Source: CAD feature listing. Evaluate the final solid. Frame: model axes, mm. Face numbers are marked on the shaded views. A direction names the side the tool comes from. Round coordinates to 2 decimals unless told otherwise and drop trailing zeros. Loops run counter-clockwise (first coordinate to the right, second up) from the corner with the lowest first, then second, coordinate; pieces in that order, holes last. Notation, with made-up numbers: (46.25, -20) - (64.25, -20) arc R17 ccw to (64.25, 1) - close; hole circle Ø1 at (-34, 28). An arc over 180 degrees is marked (long way). One line per question, with ' | ' between items. Start each with the question number.
1. Cut plane D-D (x = 0). State how many separate pieces and enclosed holes the cut face has, then the cut area to 3 significant figures.
2. Cut plane C-C (x = 4.5). Return loops of the section in (y, z) (3 decimals).
3. Ray query, line 1 (Y direction, x = 0, z = 0.2) (3 decimals); line 2 (Z direction, x = -8.5, y = -5.5); line 3 (X direction, y = -5, z = -5.25). Return the intervals inside material, ascending.
4. Cut plane B-B (z = -8.5). Return loops of the section in (x, y) (3 decimals).
5. Access query for the marked faces 5, 6 and 7. Directions: +Z, -Z, +X, -X, +Y, -Y. A direction counts if a zero-diameter tool reaches every point of the face in a straight line with its end or side. Return the directions, or none.
6. Pin query (flat end, axial travel): pin 1 (2 mm diameter, centred on y = 3, z = -6.5, fed in from -X); pin 2 (4 mm diameter, centred on x = -6, z = -10.5, fed in from -Y) (3 decimals); pin 3 (0.9 mm diameter, centred on x = -6.5, z = 0.5, fed in from +Y) (3 decimals). Return the tip coordinate at first contact, or that it passes through.
7. Mould query, pull axis Z, two halves, no side actions, for the marked faces 1, 2, 3 and 4. Classes: pulls with the +Z half, pulls with the -Z half, needs draft (parallel to the pull), parting line crosses it, or undercut.
8. Cut plane A-A (y = -2). Return loops of the section in (x, z), then the cut area to 3 significant figures.
Autodesk Inventor part; units mm, degrees
ref_plane "YZ Plane" through (0, 0, 0) normal (1, 0, 0) x (0, 1, 0)
ref_plane "XZ Plane" through (0, 0, 0) normal (0, 1, 0) x (-1, 0, 0)
ref_plane "XY Plane" through (0, 0, 0) normal (0, 0, 1) x (1, 0, 0)
sketch "Sketch1" plane through (0, 0, 0) normal (0, 0, 1) x (1, 0, 0)
  line L0 (-6.2, 6.875) -> (6.2, 6.875)
  line L1 (6.2, 6.875) -> (6.2, -6.875)
  line L2 (6.2, -6.875) -> (-6.2, -6.875)
  line L3 (-6.2, -6.875) -> (-6.2, 6.875)
  line L4 (8.8, 12.475) -> (-8.8, 12.475)
  line L5 (-11.8, 9.475) -> (-11.8, -9.475)
  line L6 (-8.8, -12.475) -> (8.8, -12.475)
  line L7 (11.8, -9.475) -> (11.8, 9.475)
  arc A0 (-8.8, 12.475) -> (-11.8, 9.475) centre (-8.8, 9.475) ccw
  arc A1 (11.8, 9.475) -> (8.8, 12.475) centre (8.8, 9.475) ccw
  arc A2 (8.8, -12.475) -> (11.8, -9.475) centre (8.8, -9.475) ccw
  arc A3 (-11.8, -9.475) -> (-8.8, -12.475) centre (-8.8, -9.475) ccw
  point P0 (0, 0)
  dimension "d0" = 12.4
  dimension "d1" = 13.75
  dimension "d2" = 5.6
  dimension "d3" = 3
  dimension "d4" = 6.875
  dimension "d5" = 6.2
  dimension "d16" = 23.6
  dimension "d17" = 24.95
extrude "Extrusion1" add sketch "Sketch1" along normal blind 0.8
sketch "Sketch3" plane through (0, 0, 0) normal (0, 0, -1) x (-1, 0, 0)
  line L0 (-6.2, -6.875) -> (-6.2, 6.875)
  line L1 (-6.2, 6.875) -> (6.2, 6.875)
  line L2 (6.2, 6.875) -> (6.2, -6.875)
  line L3 (6.2, -6.875) -> (-6.2, -6.875)
  line L4 (8.8, 12.475) -> (-8.8, 12.475)
  arc A0 (-8.8, 12.475) -> (-11.8, 9.475) centre (-8.8, 9.475) ccw
  line L5 (-11.8, 9.475) -> (-11.8, -9.475)
  arc A1 (-11.8, -9.475) -> (-8.8, -12.475) centre (-8.8, -9.475) ccw
  line L6 (-8.8, -12.475) -> (8.8, -12.475)
  arc A2 (8.8, -12.475) -> (11.8, -9.475) centre (8.8, -9.475) ccw
  line L7 (11.8, -9.475) -> (11.8, 9.475)
  arc A3 (11.8, 9.475) -> (8.8, 12.475) centre (8.8, 9.475) ccw
  line L8 (7, -7.675) -> (7, 7.675)
  line L9 (7, 7.675) -> (-7, 7.675)
  line L10 (-7, 7.675) -> (-7, -7.675)
  line L11 (-7, -7.675) -> (7, -7.675)
  point P0 (0, 0)
  dimension "d11" = 0.8
extrude "Extrusion2" add sketch "Sketch3" along normal blind 15 contours L11 L10 L9 L8
sketch "Sketch4" plane through (0, 0, -15) normal (0, 0, -1) x (-1, 0, 0)
  line L0 (7, -7.675) -> (-7, -7.675)
  line L1 (-7, -7.675) -> (-7, 7.675)
  line L2 (-7, 7.675) -> (7, 7.675)
  line L3 (7, 7.675) -> (7, -7.675)
  line L4 (8.8, 12.475) -> (-8.8, 12.475)
  arc A0 (-8.8, 12.475) -> (-11.8, 9.475) centre (-8.8, 9.475) ccw
  line L5 (-11.8, 9.475) -> (-11.8, -9.475)
  arc A1 (-11.8, -9.475) -> (-8.8, -12.475) centre (-8.8, -9.475) ccw
  line L6 (-8.8, -12.475) -> (8.8, -12.475)
  arc A2 (8.8, -12.475) -> (11.8, -9.475) centre (8.8, -9.475) ccw
  line L7 (11.8, -9.475) -> (11.8, 9.475)
  arc A3 (11.8, 9.475) -> (8.8, 12.475) centre (8.8, 9.475) ccw
  line L8 (-6.2, 6.875) -> (6.2, 6.875)
  line L9 (6.2, 6.875) -> (6.2, -6.875)
  line L10 (6.2, -6.875) -> (-6.2, -6.875)
  line L11 (-6.2, -6.875) -> (-6.2, 6.875)
  line L12 (7, -7.675) -> (7, 7.675)
  line L13 (7, 7.675) -> (-7, 7.675)
  line L14 (-7, 7.675) -> (-7, -7.675)
  line L15 (-7, -7.675) -> (7, -7.675)
  point P0 (0, 0)
extrude "Extrusion3" add sketch "Sketch4" along normal blind 0.8 contours L0 L1 L2 L3 | A3 L7 A2 L6 A1 L5 A0 L4
chamfer "Chamfer1" distance 1.1 angle 45 8 edges at (7, 0, 0) (0, -7.675, 0) (0, 7.675, 0) (-7, 0, 0) (-7, 0, -15) (0, 7.675, -15) (0, -7.675, -15) (7, 0, -15)
sketch "Sketch5" plane through (0, 0, 0.8) normal (0, 0, 1) x (1, 0, 0)
  circle A0 centre (0, 8.375) radius 0.6
  line L0 (-6.2, 6.875) -> (6.2, 6.875)
  line L1 (11.8, -9.475) -> (11.8, 9.475)
  line L2 (-11.8, 9.475) -> (-11.8, -9.475)
  line L3 (6.2, 6.875) -> (6.2, -6.875)
  line L4 (6.2, -6.875) -> (-6.2, -6.875)
  line L5 (-6.2, -6.875) -> (-6.2, 6.875)
  line L6 (-6.2, 6.875) -> (6.2, 6.875)
  line L7 (8.8, 12.475) -> (-8.8, 12.475)
  arc A1 (-8.8, 12.475) -> (-11.8, 9.475) centre (-8.8, 9.475) ccw
  line L8 (-11.8, 9.475) -> (-11.8, -9.475)
  arc A2 (-11.8, -9.475) -> (-8.8, -12.475) centre (-8.8, -9.475) ccw
  line L9 (-8.8, -12.475) -> (8.8, -12.475)
  arc A3 (8.8, -12.475) -> (11.8, -9.475) centre (8.8, -9.475) ccw
  line L10 (11.8, -9.475) -> (11.8, 9.475)
  arc A4 (11.8, 9.475) -> (8.8, 12.475) centre (8.8, 9.475) ccw
  line L11 (-8.8, 12.475) -> (8.8, 12.475)
  line L12 (3, 12.475) -> (-3, 12.475)
  line L13 (-3, 12.475) -> (-3, 19.475)
  line L14 (-3, 19.475) -> (3, 19.475)
  line L15 (3, 19.475) -> (3, 12.475)
  circle A5 centre (0, 11.375) radius 0.6
  circle A6 centre (0, 14.375) radius 0.6
  circle A7 centre (0, 17.375) radius 0.6
  point P0 (0, 0)
  dimension "d21" = 1.2
  dimension "d22" = 1.5
  dimension "d23" = 11.8
  dimension "d24" = 23.6
  dimension "d27" = 6
  dimension "d28" = 7
  dimension "d29" = 8.8
  dimension "d32" = 3
extrude "Extrusion4" add sketch "Sketch5" against normal up to surface (0.8 mm away) contours L7 L13 L14 L15
chamfer "Chamfer2" distance 2 angle 45 2 edges at (-3, 12.475, 0.4) (3, 12.475, 0.4)
extrude "Extrusion5" cut sketch "Sketch5" against normal blind 10 contours A0 | A5
fillet "Fillet1" radius 1 2 edges at (-3, 19.475, 0.4) (3, 19.475, 0.4)
equation "\"d23\" = 0.5 * d24"
equation "\"d29\" = -0.5 * d27 + 0.5 * d24"
properties part number "3DP_ABS_Electromagnet_Coil_Holder" material "ABS Plastic"
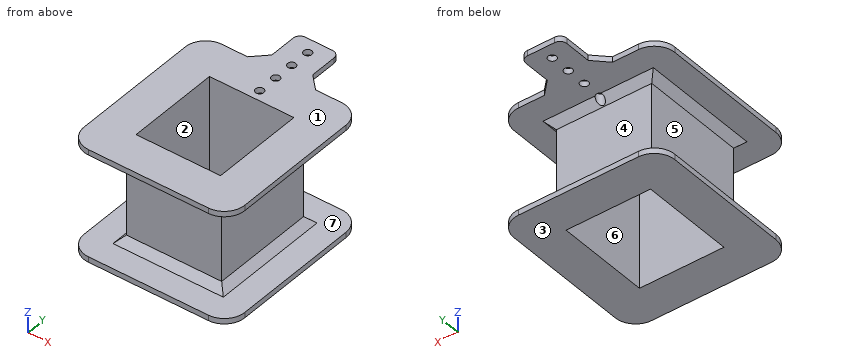
Answers follow:
1) separate pieces: 6 | enclosed holes: 0 | area: 45.6 mm2
2) outline: (-12.475, -15.8) - (-6.875, -15.8) - (-6.875, 0.8) - (-12.475, 0.8) - (-12.475, 0) - (-8.775, 0) - (-7.675, -1.1) - (-7.675, -13.9) - (-8.775, -15) - (-12.475, -15) - close; (6.875, -15.8) - (12.475, -15.8) - (12.475, -15) - (8.775, -15) - (7.675, -13.9) - (7.675, -1.1) - (8.775, 0) - (12.975, 0) - (12.975, 0.8) - (6.875, 0.8) - close
3) line 1: y = -12.475 to -6.875, 6.875 to 7.775, 8.975 to 10.775, 11.975 to 13.775, 14.975 to 16.775, 17.975 to 19.475 | line 2: z = -15.8 to -15, 0 to 0.8 | line 3: x = -7 to -6.2, 6.2 to 7
4) outline: (-7, -7.675) - (7, -7.675) - (7, 7.675) - (-7, 7.675) - close; hole (-6.2, -6.875) - (6.2, -6.875) - (6.2, 6.875) - (-6.2, 6.875) - close
5) face 5: -X, +Y, -Y | face 6: +Z, -Z | face 7: none
6) pin 1: stops at x = -7 | pin 2: stops at y = -7.675 | pin 3: stops at y = 12.475
7) face 1: pulls with the +Z half | face 2: needs draft | face 3: pulls with the -Z half | face 4: undercut
8) outline: (-11.8, -15.8) - (-6.2, -15.8) - (-6.2, 0.8) - (-11.8, 0.8) - (-11.8, 0) - (-8.1, 0) - (-7, -1.1) - (-7, -13.9) - (-8.1, -15) - (-11.8, -15) - close; (6.2, -15.8) - (11.8, -15.8) - (11.8, -15) - (8.1, -15) - (7, -13.9) - (7, -1.1) - (8.1, 0) - (11.8, 0) - (11.8, 0.8) - (6.2, 0.8) - close | area: 44.3 mm2
